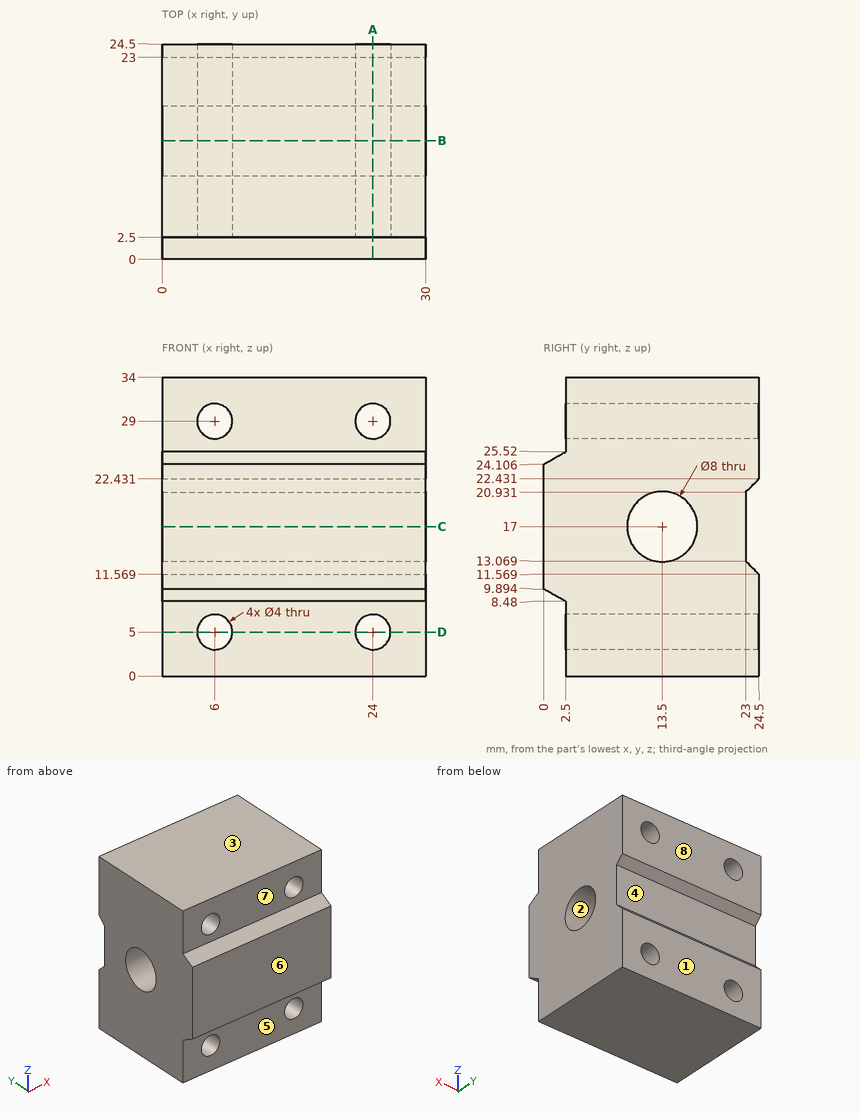
Can you work these out from the drawing? Everything is in mm from the part's minimum corner. A direction names the side the tool comes from. Round coordinates to 2 decimals unless told otherwise and drop trailing zeros. Loops run counter-clockwise (first coordinate to the right, second up) from the corner with the lowest first, then second, coordinate; pieces in that order, holes last.
1. If we section it at C-C on z = 17: Write out the boundary of the cut face in (x, y).
Answer list:
outline: (0, 0) - (30, 0) - (30, 9.5) - (0, 9.5) - close; (0, 17.5) - (30, 17.5) - (30, 23) - (0, 23) - close
2. We'd pull the mould along Z, two halves only. Please class the marked faces 1, 2 and 3: +Z half, -Z half, draft (parallel to the pull), parting line (faces both ways), or undercut.
Answer list:
face 1: draft
face 2: undercut
face 3: +Z half
3. If I drill on line 1 along X through (y, z) = (7.5, 29); line 2 along Z through (x, y) = (6, 8); line 3 along Z through (x, y) = (24, 13.75), over which ranges is the centre line in solid material (lowest first)?
Answer list:
line 1: x = 0 to 4, 8 to 22, 26 to 30
line 2: z = 0 to 3, 7 to 27, 31 to 34
line 3: z = 0 to 3, 7 to 13.01, 20.99 to 27, 31 to 34
4. For P1, Ø4, axis at x = 20, z = 2.5, coming from the -Y side; P2, Ø6.5, axis at x = 8, z = 18, coming from the +Y side, each with a flat end and sliding along its axis, tell me the tip position at first contact or that it passes through.
Answer list:
P1: stops at y = 2.5
P2: stops at y = 23.32
5. Which directions (+Z, -Z, +X, -X, +Y, -Y) give clear straight access to the entire face, cutting with the end or side of a thin tool? Please do the marked faces 4, 5, 6, 7 and 8.
Answer list:
face 4: +X, -X, +Y
face 5: -Z, +X, -X, -Y
face 6: +Z, -Z, +X, -X, -Y
face 7: +Z, +X, -X, -Y
face 8: +Z, -Z, +X, -X, +Y
6. If we section it at D-D on z = 5: Write out the boundary of the cut face in (x, y).
Answer list:
outline: (0, 2.5) - (4, 2.5) - (4, 24.5) - (0, 24.5) - close; (8, 2.5) - (22, 2.5) - (22, 24.5) - (8, 24.5) - close; (26, 2.5) - (30, 2.5) - (30, 24.5) - (26, 24.5) - close
7. If we section it at B-B on y = 13.5: Write out the boundary of the cut face in (x, z), plus the area to 3 significant figures.
Answer list:
outline: (0, 0) - (30, 0) - (30, 13) - (0, 13) - close; (0, 21) - (30, 21) - (30, 34) - (0, 34) - close; hole circle Ø4 at (6, 5); hole circle Ø4 at (6, 29); hole circle Ø4 at (24, 5); hole circle Ø4 at (24, 29)
area: 730 mm2
8. If we section it at A-A on x = 24: Count the separate pieces of the cut face and the enclosed holes in it, plus the area to 3 significant figures.
Answer list:
separate pieces: 3
enclosed holes: 1
area: 547 mm2
